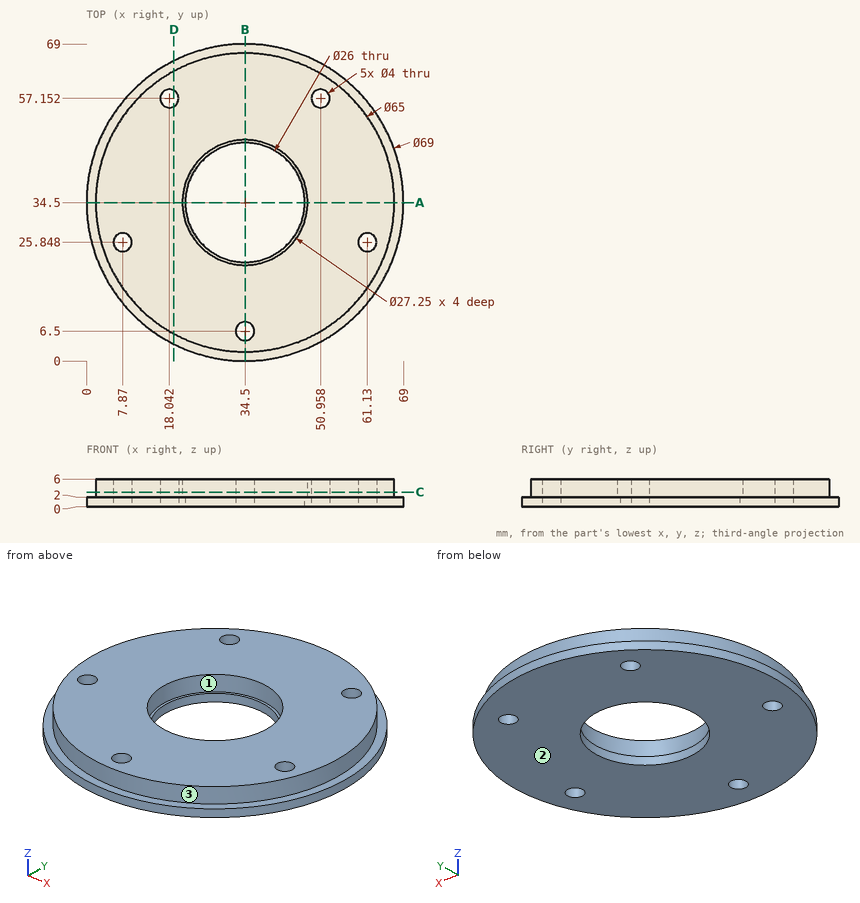
Check sheet for the drawn part. Datum: minimum x, y, z corner. Units: mm. Give positions to 0.01 mm unless a question says otherwise; leave off trailing zeros. Write each loop counter-clockwise with the first axis right and the second up, starting at its lowest first coordinate (ties: lowest second). Pieces come first, ordered by that corner, then holes. Notation, with made-up numbers: M -38,51 L -13,51 A23 cw -13,74 Z; hole C 86.5,14 d1. An arc over 180 degrees is marked long. Write item = value, one per line.
(1) Sectioned sample at A-A (y = 34.5). Record the cut outline in (x, z) (1 decimal).
Found:
outline = M 0,0 L 21.5,0 L 21.5,2 L 20.9,2 L 20.9,6 L 2,6 L 2,2 L 0,2 Z; M 47.5,0 L 69,0 L 69,2 L 67,2 L 67,6 L 48.1,6 L 48.1,2 L 47.5,2 Z
(2) Draft check along Y on the marked faces 1, 2 and 3. Enter one of: released by +Y, released by -Y, zero draft, split by the parting line, or undercut.
Found:
face_1 = undercut
face_2 = zero draft
face_3 = split by the parting line
(3) Go/stop test with flat-tipped pins: pin 1 Ø1 at (x, z) = (16.5, 3) entering from -Y (1 decimal); pin 2 Ø3 at (x, y) = (50.96, 57.15) entering from -Z; pin 3 Ø3 at (y, z) = (48, 5) entering from -X. Record where each tip stops, or that it passes through.
Found:
pin_1 = 7.1
pin_2 = through
pin_3 = 4.3
(4) Sectioned sample at B-B (x = 34.5). Record the cut outline in (y, z) (1 decimal).
Found:
outline = M 0,0 L 4.5,0 L 4.5,6 L 2,6 L 2,2 L 0,2 Z; M 8.5,0 L 21.5,0 L 21.5,2 L 20.9,2 L 20.9,6 L 8.5,6 Z; M 47.5,0 L 69,0 L 69,2 L 67,2 L 67,6 L 48.1,6 L 48.1,2 L 47.5,2 Z
(5) Sectioned sample at C-C (z = 3.15). Give the number of separate pieces and of enclosed holes in the cut face, then the cut area to 3 significant figures.
Found:
separate_pieces = 1
enclosed_holes = 6
area = 2,670 mm2
(6) Sectioned sample at D-D (x = 19). Record the cut outline in (y, z) (1 decimal).
Found:
outline = M 3.7,0 L 55.4,0 L 55.4,6 L 5.9,6 L 5.9,2 L 3.7,2 Z; M 58.9,0 L 65.3,0 L 65.3,2 L 63.1,2 L 63.1,6 L 58.9,6 Z
(7) Material ranges on line 1 (Y direction, x = 34.5, z = 1.45); line 2 (X direction, y = 27, z = 5.05) (1 decimal); line 3 (X direction, y = 27.5, z = 1.85) (1 decimal), recorded low to high.
Found:
line_1 = 0 to 4.5, 8.5 to 21.5, 47.5 to 69
line_2 = 2.9 to 6.2, 9.5 to 23.1, 45.9 to 59.5, 62.8 to 66.1
line_3 = 0.7 to 6.7, 9 to 23.5, 45.5 to 60, 62.3 to 68.3
